Can you work these out from the model? Positions are in its coordinate system, mm. Round coordinates to 2 decimals unless told otherwise and drop trailing zeros. Write each loop counter-clockwise with the first axis right and the second up, starting at its lowest first coordinate (ties: lowest second). Pieces come first, ordered by that corner, then holes. Notation, with made-up numbers: (73.5, 54.25) -> (102.5, 54.25) arc R34 ccw to (102.5, 92.25) -> close; hole circle Ø6 at (14.25, -39). An arc over 180 degrees is marked (long way). Write item = value, one per line. Start each with the question number.
1) I'm going to push flat-ended pins straight in: pin 1 (0.9 mm diameter, centred on x = 14.5, z = 2, fed in from -Y); pin 2 (0.8 mm diameter, centred on y = 66, z = 1, fed in from -X); pin 3 (0.8 mm diameter, centred on y = -1.5, z = 1.5, fed in from +X). Where does each tip first touch, or does it pass through?
2) Imagine slicing it at A-A, the plane z = 1.2. Please give me the cut outline in (x, y).
3) Imagine slicing it at C-C, the plane y = 15.5. Please give me the cut outline in (x, z).
4) If I drill on line 1 (Y direction, x = 11.25, z = 1.3); line 2 (Y direction, x = 9.5, z = 0.35); line 3 (X direction, y = 14.5, z = 0.6), over which ranges is the centre line in solid material (lowest first)?
5) Imagine slicing it at B-B, the plane x = 4. Please give me the cut outline in (y, z), then the cut area to 3 significant figures.
Autodesk Inventor part; units mm, degrees
ref_plane "YZ Plane" through (0, 0, 0) normal (1, 0, 0) x (0, 1, 0)
ref_plane "XZ Plane" through (0, 0, 0) normal (0, 1, 0) x (-1, 0, 0)
ref_plane "XY Plane" through (0, 0, 0) normal (0, 0, 1) x (1, 0, 0)
sketch "Sketch1" plane through (0, 0, 0) normal (0, 0, 1) x (1, 0, 0)
  line L0 (0, 0) -> (17, 0)
  line L1 (17, 0) -> (17, 65)
  line L2 (17, 65) -> (0, 65)
  line L3 (0, 65) -> (0, 0)
  dimension "d0" = 17
  dimension "d1" = 65
  dimension "d2" = 17
extrude "Extrusion1" add sketch "Sketch1" along normal blind 3
sketch "Sketch2" plane through (0, 0, 3) normal (0, 0, 1) x (1, 0, 0)
  line L0 (0, 0) -> (17, 0)
  line L1 (8.5, 0) -> (8.5, 11)
  line L2 (8.5, 11) -> (14.5, 11)
  line L3 (14.5, 11) -> (14.5, 20)
  line L4 (14.5, 20) -> (2.5, 20)
  line L5 (2.5, 20) -> (2.5, 11)
  line L6 (2.5, 11) -> (8.5, 11)
  dimension "d5" = 11
  dimension "d6" = 6
  dimension "d7" = 9
  dimension "d8" = 12
  dimension "d9" = 9
extrude "Extrusion2" cut sketch "Sketch2" against normal blind 16.05
sketch "Sketch3" plane through (0, 0, 0) normal (0, -1, 0) x (1, 0, 0)
  line L0 (0, 0) -> (0, 3)
  line L1 (0, 1.5) -> (17, 1.5)
  line L2 (17, 0) -> (17, 3)
  line L3 (17, 3) -> (0, 3)
  line L4 (8.5, 3) -> (8.5, 0)
  line L5 (17, 0) -> (0, 0)
  line L6 (8.5, 1.5) -> (6.5, 1.5)
  line L7 (6.5, 1.5) -> (6.5, 3)
  line L8 (8.5, 1.5) -> (10.5, 1.5)
  line L9 (10.5, 1.5) -> (10.5, 0)
  line L10 (6.5, 3) -> (10.5, 3)
  line L11 (10.5, 3) -> (10.5, 0)
  line L12 (10.5, 0) -> (6.5, 0)
  line L13 (6.5, 0) -> (6.5, 3)
  dimension "d12" = 2
  dimension "d13" = 1.5
  dimension "d14" = 2
  dimension "d15" = 1.5
extrude "Extrusion3" add sketch "Sketch3" along normal blind 2.7 contours L13 L1 L4 L5 | L7 L3 L4 L1 | L4 L1 L9 L5 | L4 L3 L11 L1
extrude "Extrusion4" add sketch "Sketch3" against normal blind 2.7 from surface at -65 contours L13 L1 L4 L5 | L7 L3 L4 L1 | L4 L1 L9 L5 | L4 L3 L11 L1
properties part number "carcasa_piezaRadio_agujero_3.0"
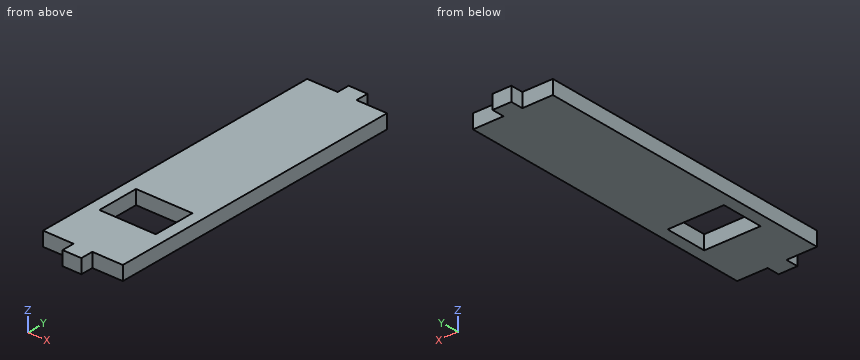
Reported:
q1.pin_1 = 0
q1.pin_2 = 6.5
q1.pin_3 = 10.5
q2.outline = (0, 0) -> (6.5, 0) -> (6.5, -2.7) -> (10.5, -2.7) -> (10.5, 0) -> (17, 0) -> (17, 65) -> (10.5, 65) -> (10.5, 67.7) -> (6.5, 67.7) -> (6.5, 65) -> (0, 65) -> close; hole (2.5, 11) -> (14.5, 11) -> (14.5, 20) -> (2.5, 20) -> close
q3.outline = (0, 0) -> (2.5, 0) -> (2.5, 3) -> (0, 3) -> close; (14.5, 0) -> (17, 0) -> (17, 3) -> (14.5, 3) -> close
q4.line_1 = 0 to 11, 20 to 65
q4.line_2 = -2.7 to 11, 20 to 67.7
q4.line_3 = 0 to 2.5, 14.5 to 17
q5.outline = (0, 0) -> (11, 0) -> (11, 3) -> (0, 3) -> close; (20, 0) -> (65, 0) -> (65, 3) -> (20, 3) -> close
q5.area = 168 mm²
